Can you work these out from the model? Positions are in its coordinate system, mm. Face numbers are marked on the shaded views. A direction names the side the tool comes from. Coordinates: 2 decimals unless noted, no trailing zeros. Order: outer loops, then holes, each group sorted by start corner. A loop starts at its lowest first (then second) coordinate and runs counter-clockwise, first axis right, second up. Notation, with made-up numbers: (27.25, -40) -> (64.25, -40) arc R19 ccw to (64.25, -9) -> close; hole circle Ø11 at (-32.5, 80). An arc over 180 degrees is marked (long way). Use a Markdown table: item, result. Add a question column.
1. For the marked faces 1 and 2, which set-ups out of +Z, -Z, +X, -X, +Y, -Y let a thin tool reach every point of the face, with its end or its side?
2. Suppose I cut it at A-A, the plane z = 31.5. List the corners of the cut face in (x, y) for me.
3. Suppose I cut it at D-D, the plane z = -21. List the corners of the cut face in (x, y) for me.
4. If I drill on line 1 along Y through (x, z) = (10, 28.5); line 2 along Y through (x, z) = (9.5, 36); line 3 along Z through (x, y) = (2, -9.5), over which ranges is the centre line in solid material (lowest first)? Write a range as from..to.
5. Suppose I cut it at C-C, the plane x = 0. List the corners of the cut face in (y, z) for me, then the cut area to 3 significant figures.
6. Suppose I cut it at B-B, the plane y = 0. List the corners of the cut face in (x, z) for me.
7. For pin 1 Ø5 at (y, z) = (-6, 21.5) entering from +X; pin 2 Ø5 at (x, z) = (11.5, 30) entering from -Y; pin 3 Ø3.5 at (x, y) = (10.5, -9.5) entering from +Z, each with a flat end and sliding along its axis, tell me the tip position at first contact or that it passes through.
```python
from build123d import *

# Parameters (mm, degrees)
SKETCH1_R           = 18
SKETCH1_R_2         = 1.5
GEARBOX_DEPTH       = 38.5
SKETCH3_R           = 4
BOSS_EXTRUDE2_DEPTH = 21.3
SKETCH4_W           = 5.291502622
SKETCH4_H           = 1
CUT_EXTRUDE1_DEPTH  = 15
FILLET1_R           = 1
SKETCH5_R           = 11
BOSS_EXTRUDE3_DEPTH = 1


with BuildPart() as part:
    # Sketch1 → GearBox (new body)
    with BuildSketch(Plane.XY):
        Circle(SKETCH1_R)
        with Locations((-10, 10)):
            Circle(SKETCH1_R_2, mode=Mode.SUBTRACT)
        with Locations((10, 10)):
            Circle(SKETCH1_R_2, mode=Mode.SUBTRACT)
        with Locations((10, -10)):
            Circle(SKETCH1_R_2, mode=Mode.SUBTRACT)
        with Locations((-10, -10)):
            Circle(SKETCH1_R_2, mode=Mode.SUBTRACT)
    extrude(amount=GEARBOX_DEPTH)

    # Sketch2 → Motor (revolve)
    with BuildSketch(Plane(origin=(0, 0, 0), x_dir=(0, 0, -1), z_dir=(1, 0, 0)), mode=Mode.PRIVATE) as motor_sk:
        with BuildLine():
            Line((0, 0), (57.5, 0))
            Line((57.5, 0), (57.5, 17.35))
            ThreePointArc((57.5, 17.35), (57.119238816, 18.269238816), (56.2, 18.65))
            Line((56.2, 18.65), (2, 18.65))
            ThreePointArc((2, 18.65), (0.585786438, 18.064213562), (0, 16.65))
            Line((0, 16.65), (0, 0))
        make_face()
    revolve(motor_sk.sketch.rotate(Axis((0, 0, 1000), (0, 0, -1)), 90), axis=Axis((0, 0, 1000), (0, 0, -1)))

    # Sketch3 → Boss-Extrude2 (add)
    with BuildSketch(Plane.XY.offset(38.5)):
        Circle(SKETCH3_R)
    extrude(amount=BOSS_EXTRUDE2_DEPTH)

    # Sketch4 → Cut-Extrude1 (cut)
    with BuildSketch(Plane.XY.offset(59.8)):
        with Locations((0, 3.5)):
            Rectangle(SKETCH4_W, SKETCH4_H)
    extrude(amount=-CUT_EXTRUDE1_DEPTH, mode=Mode.SUBTRACT)

    # Fillet1
    fillet1_edges = [part.edges().sort_by_distance(p)[0] for p in [
        (-18, 0, 38.5),
    ]]
    fillet(fillet1_edges, radius=FILLET1_R)

    # Sketch5 → Boss-Extrude3 (add)
    with BuildSketch(Plane.XY.offset(38.5)):
        Circle(SKETCH5_R)
    extrude(amount=BOSS_EXTRUDE3_DEPTH)


solid = part.part
```
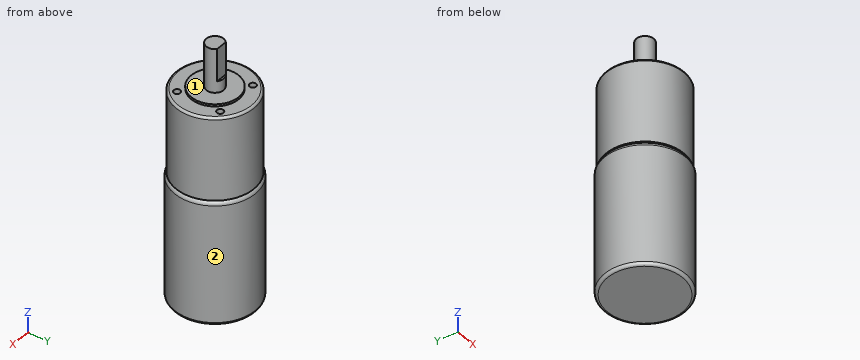
Worked out:
| question | item | result |
|---|---|---|
| 1 | face 1 | +Z |
| 1 | face 2 | +Z, -Z |
| 2 | outline | circle Ø36 at (0, 0); hole circle Ø3 at (-10, -10); hole circle Ø3 at (-10, 10); hole circle Ø3 at (10, -10); hole circle Ø3 at (10, 10) |
| 3 | outline | circle Ø37.3 at (0, 0) |
| 4 | line 1 | y = -14.97..-11.5, -8.5..8.5, 11.5..14.97 |
| 4 | line 2 | y = -15.29..-11.41, -8.59..8.59, 11.41..15.29 |
| 4 | line 3 | z = -57.5..39.5 |
| 5 | outline | (-18.65, -56.2) arc R1.3 ccw to (-17.35, -57.5) -> (17.35, -57.5) arc R1.3 ccw to (18.65, -56.2) -> (18.65, -2) arc R2 ccw to (16.65, 0) -> (18, 0) -> (18, 37.5) arc R1 ccw to (17, 38.5) -> (11, 38.5) -> (11, 39.5) -> (4, 39.5) -> (4, 44.8) -> (3, 44.8) -> (3, 59.8) -> (-4, 59.8) -> (-4, 39.5) -> (-11, 39.5) -> (-11, 38.5) -> (-17, 38.5) arc R1 ccw to (-18, 37.5) -> (-18, 0) -> (-16.65, 0) arc R2 ccw to (-18.65, -2) -> close |
| 5 | area | 3,700 mm² |
| 6 | outline | (-18.65, -56.2) arc R1.3 ccw to (-17.35, -57.5) -> (17.35, -57.5) arc R1.3 ccw to (18.65, -56.2) -> (18.65, -2) arc R2 ccw to (16.65, 0) -> (18, 0) -> (18, 37.5) arc R1 ccw to (17, 38.5) -> (11, 38.5) -> (11, 39.5) -> (4, 39.5) -> (4, 59.8) -> (-4, 59.8) -> (-4, 39.5) -> (-11, 39.5) -> (-11, 38.5) -> (-17, 38.5) arc R1 ccw to (-18, 37.5) -> (-18, 0) -> (-16.65, 0) arc R2 ccw to (-18.65, -2) -> close |
| 7 | pin 1 | stops at x = 17.66 |
| 7 | pin 2 | stops at y = -15.59 |
| 7 | pin 3 | stops at z = 38.5 |
